Geometry: final body of the model. Coordinates: model frame, mm. Face numbers are marked on the shaded views. Round coordinates to 2 decimals unless told otherwise and drop trailing zeros. Loops run counter-clockwise (first coordinate to the right, second up) from the corner with the lowest first, then second, coordinate; pieces in that order, holes last. Notation, with made-up numbers: (14, 8) - (60, 8) arc R22 cw to (60, 22) - close; hole circle Ø4 at (87.5, -3.75). An arc over 180 degrees is marked (long way). Use CSV: the item, a comma, the result in double quotes.
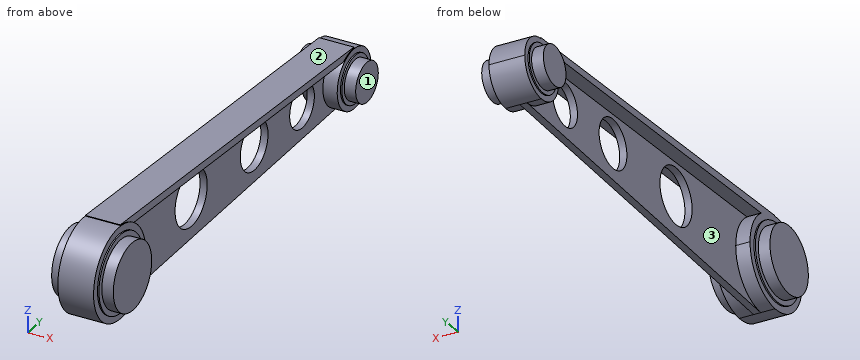
from build123d import *

# Parameters (mm, degrees)
F0_R      = 4.993118
F0_R_2    = 4.314977
F0_R_3    = 3.833909
F1_DEPTH  = 1.27
F0_R_4    = 6.876747
F0_R_5    = 4.227285
F2_DEPTH  = 3.81
F3_DEPTH  = 2.54
F5_DEPTH  = 2.54
F6_DEPTH  = 2.5146
F0_R_6    = 5.96286
F0_R_7    = 3.508795
F7_DEPTH  = 1.778
F8_DEPTH  = 3.6576
F9_DEPTH  = 4.064
F10_DEPTH = 2.794
F11_DEPTH = 2.7686
F12_DEPTH = 6.096
F13_DEPTH = 4.8514


with BuildPart() as f1:
    # F0 (on Right) → F1 (new body)
    with BuildSketch(Plane.YZ):
        with BuildLine():
            ThreePointArc((30.679518, -5.2486), (25.329293, 0.052162), (30.783797, 5.245558))
            Line((30.783797, 5.245558), (-41.582841, 8.076357))
            ThreePointArc((-41.582841, 8.076357), (-36.273612, 5.497048), (-34.123445, 0))
            ThreePointArc((-34.123445, 0), (-36.385243, -5.615502), (-41.907786, -8.095646))
            Line((-41.907786, -8.095646), (30.679518, -5.2486))
        make_face()
        with Locations((-15.587313, 0)):
            Circle(F0_R, mode=Mode.SUBTRACT)
        with Locations((3.977629, 0.031597)):
            Circle(F0_R_2, mode=Mode.SUBTRACT)
        with Locations((18.845779, 0)):
            Circle(F0_R_3, mode=Mode.SUBTRACT)
    extrude(amount=F1_DEPTH)

    # F0 (on Right) → F2 (join)
    with BuildSketch(Plane.YZ):
        with BuildLine():
            ThreePointArc((-34.123445, 0), (-36.273612, 5.497048), (-41.582841, 8.076357))
            ThreePointArc((-41.582841, 8.076357), (-50.325552, 0.162758), (-41.907786, -8.095646))
            ThreePointArc((-41.907786, -8.095646), (-36.385243, -5.615502), (-34.123445, 0))
        make_face()
        with Locations((-42.225316, 0)):
            Circle(F0_R_4, mode=Mode.SUBTRACT)
        with BuildLine():
            ThreePointArc((30.679518, -5.2486), (34.326119, -3.676155), (35.828174, 0))
            ThreePointArc((35.828174, 0), (34.362462, 3.638737), (30.783797, 5.245558))
            ThreePointArc((30.783797, 5.245558), (25.329293, 0.052162), (30.679518, -5.2486))
        make_face()
        with Locations((30.578604, 0)):
            Circle(F0_R_5, mode=Mode.SUBTRACT)
    extrude(amount=F2_DEPTH)

    # F0 (on Right) → F3 (join)
    with BuildSketch(Plane.YZ):
        with BuildLine():
            ThreePointArc((-34.123445, 0), (-36.273612, 5.497048), (-41.582841, 8.076357))
            ThreePointArc((-41.582841, 8.076357), (-50.325552, 0.162758), (-41.907786, -8.095646))
            ThreePointArc((-41.907786, -8.095646), (-36.385243, -5.615502), (-34.123445, 0))
        make_face()
        with Locations((-42.225316, 0)):
            Circle(F0_R_4, mode=Mode.SUBTRACT)
        with BuildLine():
            ThreePointArc((30.679518, -5.2486), (34.326119, -3.676155), (35.828174, 0))
            ThreePointArc((35.828174, 0), (34.362462, 3.638737), (30.783797, 5.245558))
            ThreePointArc((30.783797, 5.245558), (25.329293, 0.052162), (30.679518, -5.2486))
        make_face()
        with Locations((30.578604, 0)):
            Circle(F0_R_5, mode=Mode.SUBTRACT)
    extrude(amount=-F3_DEPTH)

    # F4 (on Right) → F5 (join)
    with BuildSketch(Plane.YZ):
        Polygon((30.701259, 4.202033), (30.785728, 5.408032), (-41.789994, 8.186051), (-41.789994, 6.797041), align=None)
    extrude(amount=-F5_DEPTH)

    # F4 (on Right) → F6 (join)
    with BuildSketch(Plane.YZ):
        Polygon((30.701259, 4.202033), (30.785728, 5.408032), (-41.789994, 8.186051), (-41.789994, 6.797041), align=None)
    extrude(amount=-F6_DEPTH)

    # F0 (on Right) → F7 (join)
    with BuildSketch(Plane.YZ):
        with Locations((-42.225316, 0)):
            Circle(F0_R_4)
        with Locations((-42.225316, 0)):
            Circle(F0_R_6, mode=Mode.SUBTRACT)
        with Locations((30.578604, 0)):
            Circle(F0_R_5)
        with Locations((30.578604, 0)):
            Circle(F0_R_7, mode=Mode.SUBTRACT)
    extrude(amount=F7_DEPTH)

    # F4 (on Right) → F8 (join)
    with BuildSketch(Plane.YZ):
        Polygon((30.701259, 4.202033), (30.785728, 5.408032), (-41.789994, 8.186051), (-41.789994, 6.797041), align=None)
    extrude(amount=F8_DEPTH)

    # F0 (on Right) → F9 (join)
    with BuildSketch(Plane.YZ):
        with Locations((30.578604, 0)):
            Circle(F0_R_5)
        with Locations((30.578604, 0)):
            Circle(F0_R_7, mode=Mode.SUBTRACT)
        with Locations((-42.225316, 0)):
            Circle(F0_R_4)
        with Locations((-42.225316, 0)):
            Circle(F0_R_6, mode=Mode.SUBTRACT)
    extrude(amount=F9_DEPTH)

    # F0 (on Right) → F10 (join)
    with BuildSketch(Plane.YZ):
        with Locations((-42.225316, 0)):
            Circle(F0_R_4)
        with Locations((-42.225316, 0)):
            Circle(F0_R_6, mode=Mode.SUBTRACT)
    extrude(amount=-F10_DEPTH)

    # F0 (on Right) → F11 (join)
    with BuildSketch(Plane.YZ):
        with Locations((30.578604, 0)):
            Circle(F0_R_5)
        with Locations((30.578604, 0)):
            Circle(F0_R_7, mode=Mode.SUBTRACT)
    extrude(amount=-F11_DEPTH)

    # F0 (on Right) → F12 (join)
    with BuildSketch(Plane.YZ):
        with Locations((-42.225316, 0)):
            Circle(F0_R_6)
        with Locations((30.578604, 0)):
            Circle(F0_R_7)
    extrude(amount=F12_DEPTH)

    # F0 (on Right) → F13 (join)
    with BuildSketch(Plane.YZ):
        with Locations((30.578604, 0)):
            Circle(F0_R_7)
        with Locations((-42.225316, 0)):
            Circle(F0_R_6)
    extrude(amount=-F13_DEPTH)


solid = f1.part
Item 1: Mould query, pull axis Y, two halves, no side actions, for the marked faces 1, 2 and 3. Classes: released by +Y, released by -Y, zero draft, split by the parting line, or undercut.
Final values:
face 1,"zero draft"
face 2,"released by +Y"
face 3,"undercut"
Item 2: Section D-D on y = -26. Return the cut outline in (x, z), plus the area to 3 significant figures.
Final values:
outline,"(-2.54, 6.23) - (0, 6.23) - (0, -7.47) - (1.27, -7.47) - (1.27, 6.23) - (3.66, 6.23) - (3.66, 7.58) - (-2.54, 7.58) - close"
area,"25.8 mm²"
Item 3: Section A-A on y = 16. Return the cut outline in (x, z), plus the area to 3 significant figures.
Final values:
outline,"(-2.54, 4.73) - (0, 4.73) - (0, 2.57) - (1.27, 2.57) - (1.27, 4.73) - (3.66, 4.73) - (3.66, 5.97) - (-2.54, 5.97) - close; (0, -5.82) - (1.27, -5.82) - (1.27, -2.57) - (0, -2.57) - close"
area,"14.6 mm²"
Item 4: Pin query (flat end, axial travel): P1, Ø2, axis at x = 4.5, y = 22, coming from the +Z side; P2, Ø1.5, axis at x = 2.5, z = 2, coming from the -Y side; P3, Ø1.5, axis at x = 2.5, y = -8, coming from the -Z side. Return the tip coordinate at first contact, or that it passes through.
Final values:
P1,"stops at z = 5.76"
P2,"stops at y = -50.23"
P3,"stops at z = 5.56"
Item 5: Section C-C on z = 2.75. Give the number of separate pieces and of enclosed holes in the cut face, plus the area to 3 significant figures.
Final values:
separate pieces,"4"
enclosed holes,"0"
area,"276 mm²"
Item 6: Material intervals for line 1 (X direction, y = -28, z = -5.5); line 2 (Y direction, x = 3.25, z = -2.25); line 3 (Y direction, x = 1.5, z = 2), sorted ascending.
Final values:
line 1,"x = 0 to 1.27"
line 2,"y = -50.01 to -34.44, 25.84 to 35.32"
line 3,"y = -50.08 to -34.37, 25.72 to 35.43"
Item 7: Section B-B on y = -3.5. Return the cut outline in (x, z), plus the area to 3 significant figures.
Final values:
outline,"(-2.54, 5.43) - (0, 5.43) - (0, -6.59) - (1.27, -6.59) - (1.27, 5.43) - (3.66, 5.43) - (3.66, 6.72) - (-2.54, 6.72) - close"
area,"23.3 mm²"
